Can you work these out from the drawing? Everything is in mm from the part's minimum corner. A direction names the side the tool comes from. Give positions to 0.01 mm unless a question says otherwise; leave off trailing zeros. Loops run counter-clockwise (first coordinate to the right, second up) from the corner with the lowest first, then second, coordinate; pieces in that order, holes last. Notation, with made-up numbers: (-37.5, 75.5) - (10.5, 75.5) arc R20 cw to (10.5, 89.5) - close; hole circle Ø9 at (5.5, 58). An arc over 180 degrees is marked (long way). One line per item, written item: value. Start each with the question number.
Q1. I want a section at C-C (x = 9.75). Please give me the cut outline in (y, z).
Q2. I'm going to push flat-ended pins straight in: P1, Ø2.5, axis at x = 37.5, y = 10.5, coming from the -Z side; P2, Ø2.5, axis at x = 11, y = 10.5, coming from the +Z side; P3, Ø3, axis at y = 11.5, z = 15, coming from the +X side. Where does each tip first touch, or does it pass through?
Q3. I want a section at A-A (y = 10.5). Please give me the cut outline in (x, z).
Q4. If I drill on line 1 (Y direction, x = 37.5, z = 7); line 2 (Y direction, x = 37.5, z = 14.7); line 3 (X direction, y = 12.25, z = 4.25), over which ranges is the centre line in solid material (lowest first)? Write a range as from..to.
Q5. For the marked faces 4 and 5, which set-ups out of +Z, -Z, +X, -X, +Y, -Y let a thin tool reach every point of the face, with its end or its side?
Q6. I want a section at B-B (z = 5.75). Please give me the cut outline in (x, y).
Q7. If we mould it in two halves opening along Y, with no side actions, what happens to the marked faces 1, 2 and 3? For each: released by +Y, released by -Y, zero draft, split by the parting line, or undercut.
Q8. I want a section at D-D (y = 7.5). Please give me the cut outline in (x, z).
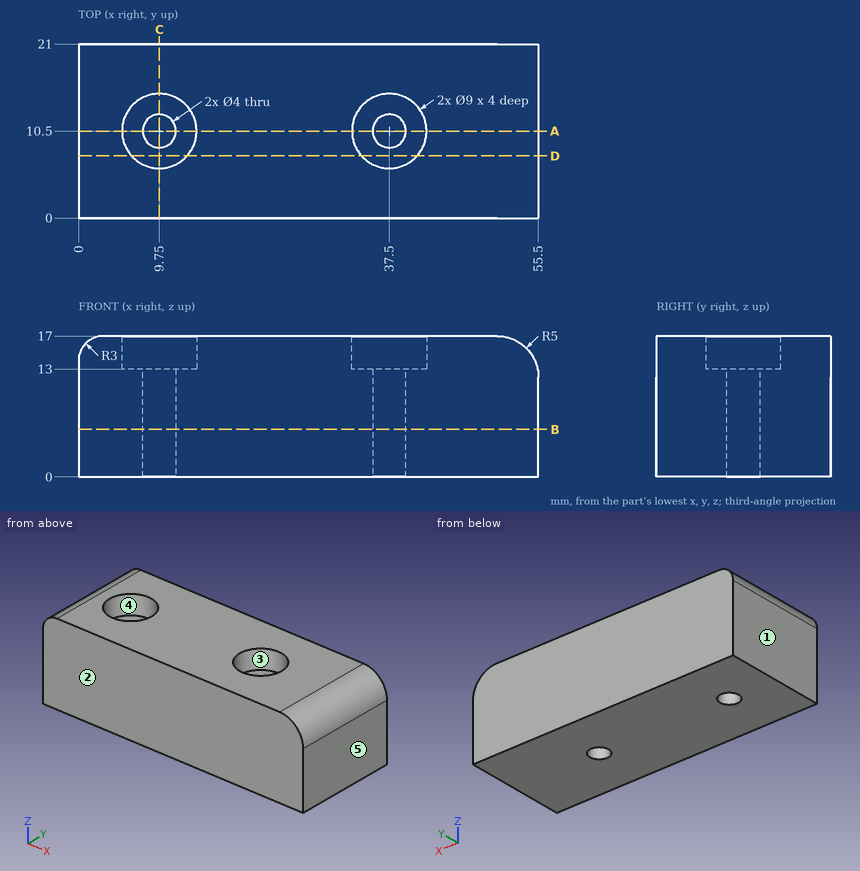
Worked answers:
1. outline: (0, 0) - (8.5, 0) - (8.5, 13) - (6, 13) - (6, 17) - (0, 17) - close; (12.5, 0) - (21, 0) - (21, 17) - (15, 17) - (15, 13) - (12.5, 13) - close
2. P1: passes through
2. P2: stops at z = 13
2. P3: stops at x = 55.27
3. outline: (0, 0) - (7.75, 0) - (7.75, 13) - (5.25, 13) - (5.25, 17) - (3, 17) arc R3 ccw to (0, 14) - close; (11.75, 0) - (35.5, 0) - (35.5, 13) - (33, 13) - (33, 17) - (14.25, 17) - (14.25, 13) - (11.75, 13) - close; (39.5, 0) - (55.5, 0) - (55.5, 12) arc R5 ccw to (50.5, 17) - (42, 17) - (42, 13) - (39.5, 13) - close
4. line 1: y = 0..8.5, 12.5..21
4. line 2: y = 0..6, 15..21
4. line 3: x = 0..8.78, 10.72..36.53, 38.47..55.5
5. face 4: +Z
5. face 5: +Z, -Z, +X, +Y, -Y
6. outline: (0, 0) - (55.5, 0) - (55.5, 21) - (0, 21) - close; hole circle Ø4 at (9.75, 10.5); hole circle Ø4 at (37.5, 10.5)
7. face 1: zero draft
7. face 2: released by -Y
7. face 3: undercut
8. outline: (0, 0) - (55.5, 0) - (55.5, 12) arc R5 ccw to (50.5, 17) - (40.85, 17) - (40.85, 13) - (34.15, 13) - (34.15, 17) - (13.1, 17) - (13.1, 13) - (6.4, 13) - (6.4, 17) - (3, 17) arc R3 ccw to (0, 14) - close
